Design review of the part built by this model. Coordinates are the model's own, in mm. A direction names the side the tool comes from. Coordinates: 2 decimals unless noted, no trailing zeros. Loops run counter-clockwise (first coordinate to the right, second up) from the corner with the lowest first, then second, coordinate; pieces in that order, holes last. Notation, with made-up numbers: (-7.5, -30.5) - (18.5, -30.5) arc R27 ccw to (18.5, -14.5) - close; hole circle Ø7 at (84, -22). An arc over 180 degrees is marked (long way). Answer in a Markdown table with one row per item. Add a question column.
(1) We need section C-C, the plane y = -2.5. Write out the cut boundary in (x, z).
(2) To check wall thickness, follow L1, parallel to Y at x = -13.9, z = 1.55; L2, parallel to Y at x = -5.5, z = 1.5; L3, parallel to Z at x = 4.75, y = -9.5. State the ranges of each line that lie inside material, in increasing order. Write a range as [from, to].
(3) The part is to be moulded in two halves that separate along X. For faces 1 (the face through (-16.05, -4, 2)), 2 (the face through (1.395, -12.072, -28.474)), 3 (the face through (13.62, -5.71, 4.26)), say which applies: released by +X, released by -X, zero draft, split by the parting line, or undercut.
(4) For faces 4 (the face through (-9, -9, 6.455)), 5 (the face through (-10.551, -6.693, 5.249)), 6 (the face through (-0.415, -12.072, 17.311)), list the 3-axis set-ups (+Z, -Z, +X, -X, +Y, -Y) from which the entire face can be reached by the end or side of a thin tool; tool diameter is ignored.
(5) We need section B-B, the plane y = 0. Write out the cut boundary in (x, z).
(6) We need section D-D, the plane z = -19. Write out the cut boundary in (x, y), plus the area to 3 significant figures.
(7) Clearance check with flat-ended pins moving along their axes: pin 1 (4.5 mm diameter, centred on x = 3.5, z = -21, fed in from +Y); pin 2 (6.5 mm diameter, centred on y = -8.5, z = -22, fed in from -X); pin 3 (2 mm diameter, centred on y = -12, z = 15.5, fed in from +X); pin 4 (5 mm diameter, centred on x = 12.5, y = -7.5, fed in from -Z). State where each tip first meets the part, or that it passes through.
(8) We need section A-A, the plane x = -13.9. Write out the cut boundary in (y, z), plus the area to 3 significant figures.
from build123d import *

# Parameters (mm, degrees)
SKETCH1_R                       = 1.016
BOSS_EXTRUDE1_DEPTH             = 2
SKETCH2_R                       = 4.7
BOSS_EXTRUDE2_DEPTH             = 3
BOSS_EXTRUDE5_DEPTH             = 8
BOSS_EXTRUDE6_REACH             = 45.699
BOSS_EXTRUDE6_DIRECTION_2_REACH = 45.699
SKETCH4_W                       = 22.5
SKETCH4_H                       = 14.127681706
CUT_EXTRUDE1_DEPTH              = 7
FILLET1_R                       = 0.5
SKETCH5_R                       = 2.5
BOSS_EXTRUDE7_DEPTH             = 1
SKETCH6_W                       = 5.313656685
SKETCH6_H                       = 4.599259183
SKETCH6_W_2                     = 16.163165117
SKETCH6_H_2                     = 5.344557169
CUT_EXTRUDE2_DEPTH              = 5


with BuildPart() as part:
    # Sketch1 → Boss-Extrude1 (new body)
    # profile 1 of 4: a face of its own
    with BuildSketch(Plane.XY):
        with BuildLine():
            Line((-16.05, 5.25), (-16.05, -5.25))
            ThreePointArc((-16.05, -5.25), (-15.801040764, -5.851040764), (-15.2, -6.1))
            Line((-15.2, -6.1), (-11.25, -6.1))
            Line((-11.25, -6.1), (-11.25, 6.1))
            Line((-11.25, 6.1), (-15.2, 6.1))
            ThreePointArc((-15.2, 6.1), (-15.801040764, 5.851040764), (-16.05, 5.25))
        make_face()
        with Locations((-13.9, 0)):
            Circle(SKETCH1_R, mode=Mode.SUBTRACT)
    # profile 2 of 4: a face of its own
    with BuildSketch(Plane.XY):
        with BuildLine():
            Line((16.05, 5.25), (16.05, -5.25))
            ThreePointArc((16.05, -5.25), (15.801040764, -5.851040764), (15.2, -6.1))
            Line((15.2, -6.1), (11.25, -6.1))
            Line((11.25, -6.1), (11.25, 6.094097151))
            Line((11.25, 6.094097151), (15.2, 6.1))
            ThreePointArc((15.2, 6.1), (15.801040764, 5.851040764), (16.05, 5.25))
        make_face()
        with Locations((13.9, 0)):
            Circle(SKETCH1_R, mode=Mode.SUBTRACT)
    # profile 3 of 4: a face of its own
    with BuildSketch(Plane.XY):
        with BuildLine():
            ThreePointArc((15.2, -6.1), (15.801040764, -5.851040764), (16.05, -5.25))
            Line((16.05, -5.25), (16.05, -6.1))
            Line((16.05, -6.1), (15.2, -6.1))
        make_face()
    # profile 4 of 4: a face of its own
    with BuildSketch(Plane.XY):
        with BuildLine():
            ThreePointArc((-16.05, -5.25), (-15.801040764, -5.851040764), (-15.2, -6.1))
            Line((-15.2, -6.1), (-16.05, -6.1))
            Line((-16.05, -6.1), (-16.05, -5.25))
        make_face()
    extrude(amount=BOSS_EXTRUDE1_DEPTH)

    # Sketch2 → Boss-Extrude2 (add)
    with BuildSketch(Plane.XZ.offset(6.1)):
        Polygon((16.05, 2), (11.25, 2), (11.25, 24.675592953), (-1.65, 19.952742461), (-1.65, 2), (-16.05, 2), (-16.05, 0), (-1.65, 0), (-1.65, -31.072136217), (11.25, -31.072136217), (11.25, 0), (16.05, 0), align=None)
        with Locations((4.75, -19)):
            Circle(SKETCH2_R, mode=Mode.SUBTRACT)
    extrude(amount=BOSS_EXTRUDE2_DEPTH)

    # Sketch2<3> → Boss-Extrude5 (add)
    with BuildSketch(Plane.XZ.offset(6.1)):
        with BuildLine():
            Line((11.231228015, 22.158640143), (11.25, 22.341096015))
            Line((11.25, 22.341096015), (11.25, 24.675592953))
            Line((11.25, 24.675592953), (-1.65, 19.952742461))
            Line((-1.65, 19.952742461), (-1.65, 16.43877001))
            ThreePointArc((-1.65, 16.43877001), (-0.396504625, 17.322324926), (0.97683102, 18.004871005))
            Line((0.97683102, 18.004871005), (11.231228015, 22.158640143))
        make_face()
        with BuildLine():
            ThreePointArc((4.75, -29.05), (1.349414108, -28.457193854), (-1.65, -26.74870957))
            Line((-1.65, -26.74870957), (-1.65, -31.072136217))
            Line((-1.65, -31.072136217), (11.25, -31.072136217))
            Line((11.25, -31.072136217), (11.25, -28.939719159))
            ThreePointArc((11.25, -28.939719159), (10.201434939, -29.022410808), (9.149976222, -29.05))
            Line((9.149976222, -29.05), (4.75, -29.05))
        make_face()
    extrude(amount=BOSS_EXTRUDE5_DEPTH)

    # Boss-Extrude6: up to this face of the body (flat: up to its plane)
    boss_extrude6_end = Plane(part.part.faces().sort_by_distance((16.05, -1.925, 1))[0])
    # Sketch3 → Boss-Extrude6 (add, up to the picked face)
    with BuildSketch(Plane(origin=(11.25, 0, 0), x_dir=(0, 0, -1), z_dir=(1, 0, 0)), mode=Mode.PRIVATE) as boss_extrude6_sk1:
        Polygon((-7.665828596, -9.1), (-2, -3.457464127), (-2, -9.1), align=None)
    boss_extrude6_tool1 = split(extrude(boss_extrude6_sk1.sketch, amount=BOSS_EXTRUDE6_REACH, mode=Mode.PRIVATE), bisect_by=boss_extrude6_end, keep=Keep.BOTH, mode=Mode.PRIVATE)
    add(boss_extrude6_tool1.solids().sort_by(Axis((11.25, -7.219155, 3.88861), (1, 0, 0)))[0])

    # Boss-Extrude6 direction 2: up to this face of the body (flat: up to its plane)
    boss_extrude6_direction_2_end = Plane(part.part.faces().sort_by_distance((-16.05, -1.925, 1))[0])
    # Sketch3 → Boss-Extrude6 direction 2 (add, up to the picked face)
    with BuildSketch(Plane(origin=(11.25, 0, 0), x_dir=(0, 0, -1), z_dir=(1, 0, 0)), mode=Mode.PRIVATE) as boss_extrude6_direction_2_sk1:
        Polygon((-7.665828596, -9.1), (-2, -3.457464127), (-2, -9.1), align=None)
    boss_extrude6_direction_2_tool1 = split(extrude(boss_extrude6_direction_2_sk1.sketch, amount=-BOSS_EXTRUDE6_DIRECTION_2_REACH, mode=Mode.PRIVATE), bisect_by=boss_extrude6_direction_2_end, keep=Keep.BOTH, mode=Mode.PRIVATE)
    add(boss_extrude6_direction_2_tool1.solids().sort_by(Axis((11.25, -7.219155, 3.88861), (-1, 0, 0)))[0])

    # Sketch4 → Cut-Extrude1 (cut)
    with BuildSketch(Plane(origin=(0, -6.1, 0), x_dir=(1, 0, 0), z_dir=(0, 1, 0))):
        with Locations((0, -7.063840853)):
            Rectangle(SKETCH4_W, SKETCH4_H)
    extrude(amount=CUT_EXTRUDE1_DEPTH, mode=Mode.SUBTRACT)

    # Fillet1
    fillet1_edges = [part.edges().sort_by_distance(p)[0] for p in [
        (13.65, -9.1, 7.665828596),
        (-8.85, -9.1, 7.665828596),
    ]]
    fillet(fillet1_edges, radius=FILLET1_R)

    # Sketch5 → Boss-Extrude7 (add)
    with BuildSketch(Plane.XZ.offset(9.1)):
        with BuildLine():
            Line((-1.65, 16.43877001), (-1.65, 6.455196792))
            Line((-1.65, 6.455196792), (-16.05, 6.455196792))
            Line((-16.05, 6.455196792), (-16.05, 0))
            Line((-16.05, 0), (-1.65, 0))
            Line((-1.65, 0), (-1.65, -26.74870957))
            ThreePointArc((-1.65, -26.74870957), (1.349414108, -28.457193854), (4.75, -29.05))
            Line((4.75, -29.05), (9.149976222, -29.05))
            ThreePointArc((9.149976222, -29.05), (10.201434939, -29.022410808), (11.25, -28.939719159))
            Line((11.25, -28.939719159), (11.25, 0))
            Line((11.25, 0), (16.05, 0))
            Line((16.05, 0), (16.05, 6.455196792))
            Line((16.05, 6.455196792), (11.25, 6.455196792))
            Line((11.25, 6.455196792), (11.25, 22.341096015))
            Line((11.25, 22.341096015), (11.231228015, 22.158640143))
            Line((11.231228015, 22.158640143), (0.97683102, 18.004871005))
            ThreePointArc((0.97683102, 18.004871005), (-0.396504625, 17.322324926), (-1.65, 16.43877001))
        make_face()
        with Locations((4.75, -19)):
            Circle(SKETCH5_R, mode=Mode.SUBTRACT)
    extrude(amount=BOSS_EXTRUDE7_DEPTH)

    # Sketch6 → Cut-Extrude2 (cut)
    with BuildSketch(Plane.XY.offset(6.455196792)):
        with Locations((13.906828343, -7.800370409)):
            Rectangle(SKETCH6_W, SKETCH6_H)
        with Locations((-9.731582558, -7.427721416)):
            Rectangle(SKETCH6_W_2, SKETCH6_H_2)
    extrude(amount=CUT_EXTRUDE2_DEPTH, mode=Mode.SUBTRACT)


solid = part.part
Responses:
| question | item | result |
|---|---|---|
| 1 | outline | (-16.05, 0) - (-11.25, 0) - (-11.25, 2) - (-16.05, 2) - close; (11.25, 0) - (16.05, 0) - (16.05, 2) - (11.25, 2) - close |
| 2 | L1 | y = [-10.1, -1.02], [1.02, 6.1] |
| 2 | L2 | y = [-10.1, -6.1] |
| 2 | L3 | z = [-31.07, -21.5], [-16.5, 22.3] |
| 3 | face 1 | released by -X |
| 3 | face 2 | undercut |
| 3 | face 3 | zero draft |
| 4 | face 4 | +Z, -X, +Y, -Y |
| 4 | face 5 | +Z, -X, +Y |
| 4 | face 6 | +X, -Y |
| 5 | outline | (-16.05, 0) - (-14.92, 0) - (-14.92, 2) - (-16.05, 2) - close; (-12.88, 0) - (-11.25, 0) - (-11.25, 2) - (-12.88, 2) - close; (11.25, 0) - (12.88, 0) - (12.88, 2) - (11.25, 2) - close; (14.92, 0) - (16.05, 0) - (16.05, 2) - (14.92, 2) - close |
| 6 | outline | (-1.65, -10.1) - (2.25, -10.1) - (2.25, -9.1) - (0.05, -9.1) - (0.05, -6.1) - (-1.65, -6.1) - close; (7.25, -10.1) - (11.25, -10.1) - (11.25, -6.1) - (9.45, -6.1) - (9.45, -9.1) - (7.25, -9.1) - close |
| 6 | area | 18.4 mm2 |
| 7 | pin 1 | stops at y = -9.1 |
| 7 | pin 2 | stops at x = -1.65 |
| 7 | pin 3 | stops at x = -1.58 |
| 7 | pin 4 | stops at z = -31.07 |
| 8 | outline | (-10.1, 0) - (-1.02, 0) - (-1.02, 2) - (-3.46, 2) - (-7.89, 6.46) - (-10.1, 6.46) - close; (1.02, 0) - (6.1, 0) - (6.1, 2) - (1.02, 2) - close |
| 8 | area | 48.0 mm2 |
